Build history of the part. All positions in model axes, mm. A direction names the side the tool comes from. Round coordinates to 2 decimals unless told otherwise and drop trailing zeros. Loops run counter-clockwise (first coordinate to the right, second up) from the corner with the lowest first, then second, coordinate; pieces in that order, holes last.
from build123d import *

# Parameters (mm, degrees)
BOSS_EXTRUDE1_DEPTH      = 64
BOSS_EXTRUDE1_DEPTH_BACK = 64
SKETCH1_W                = 200
SKETCH1_H                = 150
SKETCH1_W_2              = 40
SKETCH1_H_2              = 15
SHELL1_T                 = -5


with BuildPart() as part:
    # Sketch1 → Boss-Extrude1 (new, two sides: drawn at the far end of the back side and taken through both)
    with BuildSketch(Plane.XY.offset(-BOSS_EXTRUDE1_DEPTH_BACK)):
        with Locations((63.345771361, 90)):
            Rectangle(SKETCH1_W, SKETCH1_H)
        with Locations((20, 7.5)):
            Rectangle(SKETCH1_W_2, SKETCH1_H_2)
    extrude(amount=BOSS_EXTRUDE1_DEPTH + BOSS_EXTRUDE1_DEPTH_BACK)

    # Shell1
    shell1_openings = [part.faces().sort_by_distance(p)[0] for p in [
        (20, 0, 0),
    ]]
    offset(amount=SHELL1_T, openings=shell1_openings, kind=Kind.INTERSECTION)


solid = part.part
(1) Pin check, flat tips, straight feed: P1, Ø10, axis at x = 111.5, z = -46, coming from the -Y side; P2, Ø6, axis at x = 34.5, z = 4.5, coming from the -Y side; P3, Ø16.5, axis at y = 6.5, z = 9, coming from the -X side; P4, Ø10, axis at y = 9.5, z = -14.5, coming from the +X side. Stop position of each tip, or through.
Responses:
P1: stops at y = 15
P2: stops at y = 0
P3: stops at x = 0
P4: stops at x = 40
(2) Which spindle directions (+Z, -Z, +X, -X, +Y, -Y) get a long thin tool onto all of the face, cutting with end or side? Do faces 4 (the face through (40, 7, -1)), 5 (the face through (-19, 15, -1)), 6 (the face through (158.346, 89, -1)), 7 (the face through (35, 10, -1)). Say none if no direction does.
Responses:
face 4: +Z, -Z, +X, -Y
face 5: +Z, -Z, -X, -Y
face 6: none
face 7: -Y
(3) Pull direction Y, two halves, no side cores. Call faces 1 (the face through (-14, 20, -1)), 2 (the face through (4, 0, -5)), 3 (the face through (163.346, 89, -1)): +Y half, -Y half, draft (parallel to the pull), parting line (faces both ways), or undercut.
Responses:
face 1: undercut
face 2: -Y half
face 3: draft
(4) Slice it at B-B on y = 136.5. List the corners of the cut face in (x, z), plus the area to 3 significant figures.
Responses:
outline: (-36.65, -64) - (163.35, -64) - (163.35, 64) - (-36.65, 64) - close; hole (-31.65, -59) - (158.35, -59) - (158.35, 59) - (-31.65, 59) - close
area: 3,180 mm2
(5) Slice it at A-A on x = 86.5. List the corners of the cut face in (y, z).
Responses:
outline: (15, -64) - (165, -64) - (165, 64) - (15, 64) - close; hole (20, -59) - (160, -59) - (160, 59) - (20, 59) - close
(6) Probe line 1 (Z direction, x = 27, y = 25.5); line 2 (Y direction, x = 45.5, z = 25); line 3 (X direction, y = 125.5, z = -35). List the from-to ranges inside material, lowest first.
Responses:
line 1: z = -64 to -59, 59 to 64
line 2: y = 15 to 20, 160 to 165
line 3: x = -36.65 to -31.65, 158.35 to 163.35
(7) Slice it at C-C on z = -37. List the corners of the cut face in (x, y), plus the area to 3 significant figures.
Responses:
outline: (-36.65, 15) - (0, 15) - (0, 0) - (5, 0) - (5, 20) - (-31.65, 20) - (-31.65, 160) - (158.35, 160) - (158.35, 20) - (35, 20) - (35, 0) - (40, 0) - (40, 15) - (163.35, 15) - (163.35, 165) - (-36.65, 165) - close
area: 3,400 mm2
